```python
from build123d import *

# Parameters (mm, degrees)
SKETCH1_W               = 304.8
SKETCH1_H               = 76.2
BOSS_EXTRUDE1_DEPTH     = 6.35
CHAMFER1_SIZE           = 53.975
CHAMFER1_SIZE2          = 37.793701875
SKETCH2_W               = 37.973
SKETCH2_H               = 6.35
BOSS_EXTRUDE2_DEPTH     = 6.35
LPATTERN1_COUNT         = 3
LPATTERN1_PITCH         = 69.85
F_3_8_CLEARANCE_HOLE1_D = 10.0838
CUT_EXTRUDE1_DEPTH      = 7.35
FILLET1_R               = 12.7
SKETCH7_W               = 6.604
SKETCH7_H               = 38.354
CUT_EXTRUDE2_DEPTH      = 7.35
CUT_EXTRUDE3_DEPTH      = 7.35
FILLET2_R               = 6.35


with BuildPart() as part:
    # Sketch1 → Boss-Extrude1 (new body)
    with BuildSketch(Plane(origin=(0, 0, 0), x_dir=(1, 0, 0), z_dir=(0, 1, 0))):
        with Locations((-152.4, -38.1)):
            Rectangle(SKETCH1_W, SKETCH1_H)
    extrude(amount=BOSS_EXTRUDE1_DEPTH)

    # Chamfer1
    chamfer1_edges = [part.edges().sort_by_distance(p)[0] for p in [
        (0, 3.175, 76.2),
    ]]
    chamfer1_side = [part.faces().sort_by_distance(p)[0] for p in [
        (-152.4, 3.175, 76.2),
    ]]
    chamfer(chamfer1_edges, length=CHAMFER1_SIZE, length2=CHAMFER1_SIZE2, reference=chamfer1_side[0])

    # Sketch2 → Boss-Extrude2 (add)
    with BuildSketch(Plane(origin=(0, 6.35, 0), x_dir=(1, 0, 0), z_dir=(0, 1, 0))):
        with Locations((-18.9865, 3.175)):
            Rectangle(SKETCH2_W, SKETCH2_H)
    boss_extrude2 = extrude(amount=-BOSS_EXTRUDE2_DEPTH)

    # LPattern1: Boss-Extrude2 ×3
    with Locations(*[(-i * LPATTERN1_PITCH, 0, 0) for i in range(1, LPATTERN1_COUNT)]):
        add(boss_extrude2)

    # 3/8 Clearance Hole1 (through all)
    with Locations(Plane(origin=(0, 6.35, 0), x_dir=(1, 0, 0), z_dir=(0, 1, 0))):
        with Locations((-37.5406093, -38.1), (-75.6406093, -38.1), (-113.7406093, -38.1), (-151.8406093, -38.1), (-189.9406093, -38.1), (-228.0406093, -38.1)):
            Hole(F_3_8_CLEARANCE_HOLE1_D / 2)

    # Sketch6 → Cut-Extrude1 (cut, through all)
    with BuildSketch(Plane(origin=(0, 6.35, 0), x_dir=(1, 0, 0), z_dir=(0, 1, 0))):
        with BuildLine():
            Line((-244.677025408, -28.8192587), (-228.6, 0))
            Line((-228.6, 0), (-304.8, 0))
            Line((-304.8, 0), (-304.8, -76.2))
            Line((-304.8, -76.2), (-228.6, -76.2))
            Line((-228.6, -76.2), (-244.677025408, -47.3807413))
            ThreePointArc((-244.677025408, -47.3807413), (-247.0906093, -38.1), (-244.677025408, -28.8192587))
        make_face()
    extrude(amount=-CUT_EXTRUDE1_DEPTH, mode=Mode.SUBTRACT)

    # Fillet1
    fillet1_edges = [part.edges().sort_by_distance(p)[0] for p in [
        (-228.6, 3.175, 76.2),
        (-228.6, 3.175, 0),
        (0, 3.175, 38.406298125),
        (-53.975, 3.175, 76.2),
    ]]
    fillet(fillet1_edges, radius=FILLET1_R)

    # Sketch7 → Cut-Extrude2 (cut, through all)
    with BuildSketch(Plane(origin=(0, 6.35, 0), x_dir=(1, 0, 0), z_dir=(0, 1, 0))):
        with Locations((-94.6906093, -38.1)):
            Rectangle(SKETCH7_W, SKETCH7_H)
    extrude(amount=-CUT_EXTRUDE2_DEPTH, mode=Mode.SUBTRACT)

    # Sketch8 → Cut-Extrude3 (cut, through all)
    with BuildSketch(Plane(origin=(0, 6.35, 0), x_dir=(1, 0, 0), z_dir=(0, 1, 0))):
        with BuildLine():
            Line((-113.7406093, -57.15), (-228.0406093, -57.15))
            ThreePointArc((-228.0406093, -57.15), (-237.686965561, -54.527121199), (-244.677025408, -47.3807413))
            Line((-244.677025408, -47.3807413), (-232.233232947, -69.687160867))
            ThreePointArc((-232.233232947, -69.687160867), (-227.573193049, -74.451414133), (-221.142288875, -76.2))
            Line((-221.142288875, -76.2), (-101.0406093, -76.2))
            Line((-101.0406093, -76.2), (-113.7406093, -57.15))
        make_face()
        with BuildLine():
            Line((-75.6406093, -57.15), (-88.3406093, -76.2))
            Line((-88.3406093, -76.2), (-57.979294619, -76.2))
            ThreePointArc((-57.979294619, -76.2), (-54.160330965, -75.612205275), (-50.694873877, -73.903230962))
            Line((-50.694873877, -73.903230962), (-26.768780472, -57.15))
            Line((-26.768780472, -57.15), (-75.6406093, -57.15))
        make_face()
    extrude(amount=-CUT_EXTRUDE3_DEPTH, mode=Mode.SUBTRACT)

    # Fillet2
    fillet2_edges = [part.edges().sort_by_distance(p)[0] for p in [
        (-113.7406093, 3.175, 57.15),
        (-101.0406093, 3.175, 76.2),
        (-75.6406093, 3.175, 57.15),
        (-26.768780472, 3.175, 57.15),
        (-88.3406093, 3.175, 76.2),
    ]]
    fillet(fillet2_edges, radius=FILLET2_R)


solid = part.part
```
Geometry check sheet. Reference: the model listing, model coordinates, mm. A direction names the side the tool comes from. Round coordinates to 2 decimals unless told otherwise and drop trailing zeros. Write each loop counter-clockwise with the first axis right and the second up, starting at its lowest first coordinate (ties: lowest second). Pieces come first, ordered by that corner, then holes. Notation, with made-up numbers: (49.5, -3) -> (56.5, -3) arc R23 ccw to (56.5, 28) -> close; hole circle Ø6 at (9, 49.5). An arc over 180 degrees is marked (long way). Put each result on its own line as item: value.
1) Cross-section at B-B, the plane z = 36. Give the number of separate pieces and of enclosed holes in the cut face, plus the area to 3 significant figures.
Recorded:
separate pieces: 8
enclosed holes: 0
area: 1,170 mm2
2) Depth check by flat-ended pin: P1, Ø8, axis at x = -29.5, z = 29, coming from the -Y side; P2, Ø3, axis at x = -131.5, y = 3.5, coming from the -Z side; P3, Ø3, axis at x = -183, y = 3, coming from the +Z side. Enter the tip coordinate at first touch or a pass-through.
Recorded:
P1: stops at y = 0
P2: stops at z = 0
P3: stops at z = 57.15
3) Thickness scan on probe 1 along Z at (x, y) = (-152.5, 4); probe 2 along Z at (x, y) = (-54, 5.25); probe 3 along Z at (x, y) = (-39, 5.5). Record the ranges inside material, lowest first. Write a range as from..to.
Recorded:
probe 1: z = -6.35..33.1, 43.1..57.15
probe 2: z = 0..57.15
probe 3: z = 0..33.27, 42.93..57.15
4) Cross-section at C-C, the plane x = -50.5. Enter the section's corners in (y, z).
Recorded:
outline: (0, 0) -> (6.35, 0) -> (6.35, 57.15) -> (0, 57.15) -> close
5) Release check for a two-part mould opening along Z. For faces 1 (the face through (-184.904, 3.131, 37.878)), 2 (the face through (-1.396, 3.219, 37.583)), 3 (the face through (-238.54, 3.22, 17.82)) record: pulls with the +Z half, pulls with the -Z half, needs draft (parallel to the pull), parting line crosses it, or undercut.
Recorded:
face 1: undercut
face 2: pulls with the +Z half
face 3: pulls with the -Z half
6) Cross-section at A-A, the plane z = 52.5. Enter the section's corners in (x, y).
Recorded:
outline: (-240.51, 0) -> (-97.99, 0) -> (-97.99, 6.35) -> (-240.51, 6.35) -> close; (-91.39, 0) -> (-20.13, 0) -> (-20.13, 6.35) -> (-91.39, 6.35) -> close
7) Access from +Z, -Z, +X, -X, +Y, -Y to the whole of each face (thin tool, end or side, straight path). Record for faces 4 (the face through (-89, 3, -6.35)), 5 (the face through (-107.823, 3, -3)).
Recorded:
face 4: -Z, +X, -X, +Y, -Y
face 5: -Z, +Y, -Y
